Geometry: see drawing. Coordinates: mm, zero at the bounding-box minimum. A direction names the side the tool comes from. Round coordinates to 2 decimals unless told otherwise and drop trailing zeros. Write each loop counter-clockwise with the first axis right and the second up, starting at its lowest first coordinate (ties: lowest second). Pieces come first, ordered by that corner, then holes. Notation, with made-up numbers: M 41.25,-23.5 L 61.25,-23.5 A23 ccw 61.25,-7.5 Z; hole C 75.5,18 d4. An arc over 180 degrees is marked long. Use one line per item in the form item = value. Start each with the question number.
Item 1: Pin query (flat end, axial travel): pin 1 Ø4 at (y, z) = (5, 17) entering from +X; pin 2 Ø4 at (x, z) = (2, 30.5) entering from +Y; pin 3 Ø1.3 at (x, z) = (1, 15.5) entering from -Y. Return the tip coordinate at first contact, or that it passes through.
Item 2: Section query B-B (z = 5.5). Return loops of the section in (x, y), and give its area (3 significant figures).
Item 3: Pull-direction query (Z, two-part tool) for the marked faces 3 and 4; classes: pulls with the +Z half, pulls with the -Z half, needs draft (parallel to the pull), parting line crosses it, or undercut.
Item 4: Ray query, probe 1 along Y at (x, z) = (3.8, 1.15); probe 2 along Y at (x, z) = (3.8, 3); probe 3 along X at (y, z) = (1.75, 24.5). Return the intervals inside material, ascending.
Item 5: Section query C-C (x = 5.5). Return loops of the section in (y, z).
Item 6: Section query D-D (z = 27). Return loops of the section in (x, y).
Item 7: Section query A-A (x = 3.8). Return loops of the section in (y, z), and give its area (3 significant figures).
Item 8: Reachability of the marked faces 1 and 2 from +Z, -Z, +X, -X, +Y, -Y: full face, straight path, thin tool, end or side. Return the list, or none.
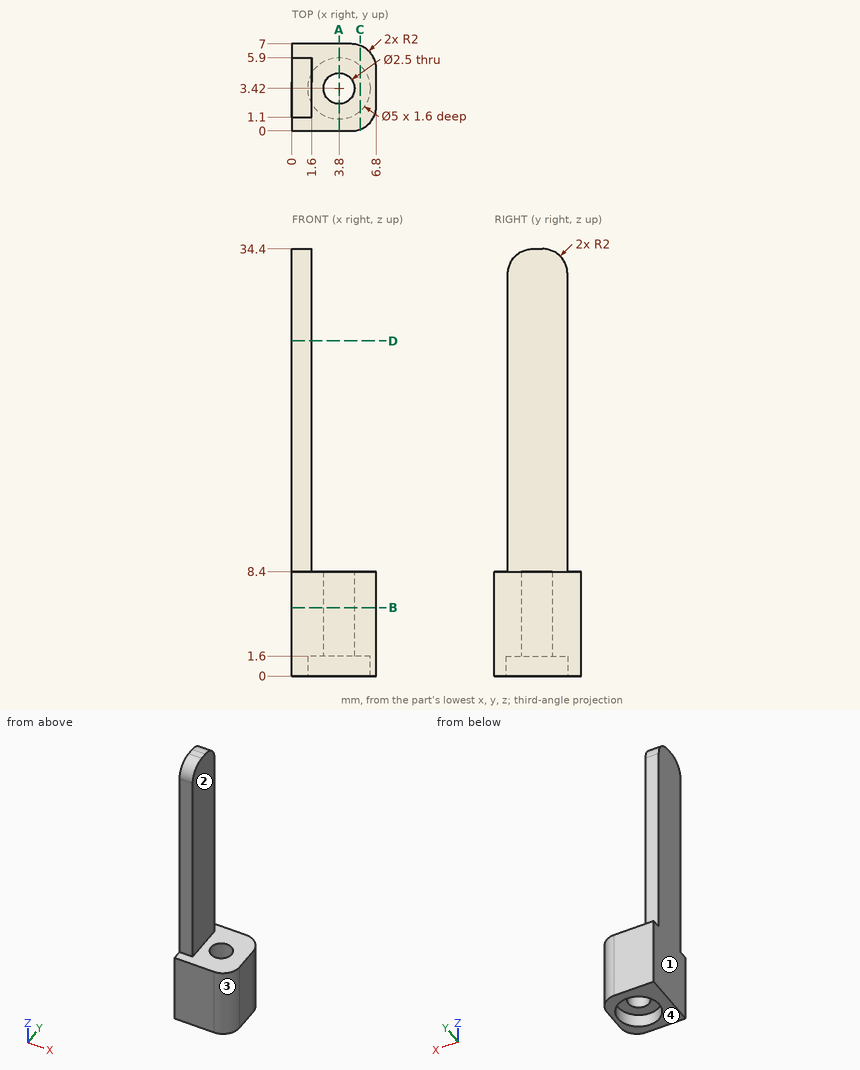
Working result:
q1.pin_1 = 1.6
q1.pin_2 = 5.9
q1.pin_3 = 1.1
q2.outline = M 0,0 L 4.8,0 A2 ccw 6.8,2 L 6.8,5 A2 ccw 4.8,7 L 0,7 Z; hole C 3.8,3.42 d2.5
q2.area = 41.0 mm²
q3.face_3 = needs draft
q3.face_4 = pulls with the -Z half
q4.probe_1 = 0 to 0.92, 5.92 to 7
q4.probe_2 = 0 to 2.17, 4.67 to 7
q4.probe_3 = 0 to 1.6
q5.outline = M 0.13,0 L 1.59,0 L 1.59,1.6 L 5.25,1.6 L 5.25,0 L 6.87,0 L 6.87,8.4 L 0.13,8.4 Z
q6.outline = M 0,1.1 L 1.6,1.1 L 1.6,5.9 L 0,5.9 Z
q7.outline = M 0,0 L 0.92,0 L 0.92,1.6 L 2.17,1.6 L 2.17,8.4 L 0,8.4 Z; M 4.67,1.6 L 5.92,1.6 L 5.92,0 L 7,0 L 7,8.4 L 4.67,8.4 Z
q7.area = 33.8 mm²
q8.face_1 = +Z, -Z, -X, +Y, -Y
q8.face_2 = +Z, +X, +Y, -Y
